from build123d import *

# Parameters (mm, degrees)
BOSS_EXTRUDE1_DEPTH   = 6.35
SKETCH2_W             = 18
SKETCH2_H             = 3
SKETCH2_W_2           = 10
SKETCH2_H_2           = 5
CUT_EXTRUDE1_DEPTH    = 148.509567486
CUT_EXTRUDE2_DEPTH    = 148.509567486
F_3_0MM_DOWEL_HOLE1_D = 3.2


with BuildPart() as part:
    # Sketch1 → Boss-Extrude1 (new body)
    with BuildSketch(Plane(origin=(0, 0, 0), x_dir=(1, 0, 0), z_dir=(0, 1, 0))):
        Polygon((64.951905284, 87.5), (-64.951905284, 87.5), (-108.253175473, 12.5), (-43.301270189, -100), (43.301270189, -100), (108.253175473, 12.5), align=None)
    extrude(amount=BOSS_EXTRUDE1_DEPTH)

    # Sketch2 → Cut-Extrude1 (cut, through all)
    with BuildSketch(Plane(origin=(0, 6.35, 0), x_dir=(1, 0, 0), z_dir=(0, 1, 0))):
        with Locations((-29, -92.2)):
            Rectangle(SKETCH2_W, SKETCH2_H)
        with Locations((29, -92.2)):
            Rectangle(SKETCH2_W, SKETCH2_H)
        Polygon((-62.146580335, 79.758965344), (-59.548504123, 78.258965344), (-68.548504123, 62.670508076), (-71.146580335, 64.170508076), align=None)
        Polygon((-97.548504123, 12.441034656), (-88.548504123, 28.029491924), (-91.146580335, 29.529491924), (-100.146580335, 13.941034656), align=None)
        Polygon((100.146580335, 13.941034656), (91.146580335, 29.529491924), (88.548504123, 28.029491924), (97.548504123, 12.441034656), align=None)
        Polygon((59.548504123, 78.258965344), (62.146580335, 79.758965344), (71.146580335, 64.170508076), (68.548504123, 62.670508076), align=None)
        with Locations((-29, -69.2)):
            Rectangle(SKETCH2_W_2, SKETCH2_H_2)
        with Locations((29, -69.2)):
            Rectangle(SKETCH2_W_2, SKETCH2_H_2)
        Polygon((79.094021451, 6.405136271), (74.094021451, 15.065390309), (69.763894432, 12.565390309), (74.763894432, 3.905136271), align=None)
        Polygon((40.763894432, 62.794863729), (45.094021451, 65.294863729), (50.094021451, 56.634609691), (45.763894432, 54.134609691), align=None)
        Polygon((-74.763894432, 3.905136271), (-69.763894432, 12.565390309), (-74.094021451, 15.065390309), (-79.094021451, 6.405136271), align=None)
        Polygon((-45.094021451, 65.294863729), (-40.763894432, 62.794863729), (-45.763894432, 54.134609691), (-50.094021451, 56.634609691), align=None)
    extrude(amount=-CUT_EXTRUDE1_DEPTH, mode=Mode.SUBTRACT)

    # Sketch4 → Cut-Extrude2 (cut, through all)
    with BuildSketch(Plane(origin=(0, 6.35, 0), x_dir=(1, 0, 0), z_dir=(0, 1, 0))):
        Polygon((35, -60.621778265), (70, 0), (35, 60.621778265), (-35, 60.621778265), (-70, 0), (-35, -60.621778265), align=None)
    extrude(amount=-CUT_EXTRUDE2_DEPTH, mode=Mode.SUBTRACT)

    # Ø3.0mm Dowel Hole1 (through all)
    with Locations(Plane(origin=(0, 6.35, 0), x_dir=(1, 0, 0), z_dir=(0, 1, 0))):
        with Locations((0, 74.060889132), (-64.138611416, -37.030444566), (64.138611416, -37.030444566)):
            Hole(F_3_0MM_DOWEL_HOLE1_D / 2)


solid = part.part
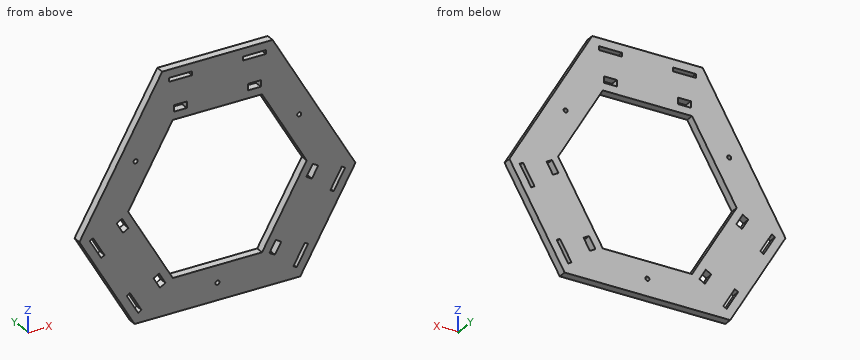
For this review, take the finished solid that the model builds, in its own axes (mm). Give positions to 0.01 mm unless a question says otherwise; leave off trailing zeros. Order: outer loops, then holes, each group sorted by start corner. A loop starts at its lowest first (then second) coordinate and runs counter-clockwise, first axis right, second up. Notation, with made-up numbers: (74.5, 42) -> (79.5, 42) arc R11 cw to (79.5, 55) -> close; hole circle Ø6 at (-34, 27). An arc over 180 degrees is marked (long way). Write item = value, one per line.
1) We need section A-A, the plane x = 9.5. Give the boundary of the cut face in (y, z), and give its area (3 significant figures).
Findings:
outline = (0, -87.5) -> (6.35, -87.5) -> (6.35, -60.62) -> (0, -60.62) -> close; (0, 60.62) -> (6.35, 60.62) -> (6.35, 100) -> (0, 100) -> close
area = 421 mm^2
2) To check wall thickness, follow L1, parallel to Z at x = 0, y = 2.5; L2, parallel to Z at x = 60.5, y = 0.75; L3, parallel to Z at x = 26, y = 3.75. State the ranges of each line that lie inside material, in increasing order. Write a range as from..to.
Findings:
L1 = -87.5..-75.66, -72.46..-60.62, 60.62..100
L2 = -87.5..-78.81, -76.61..-16.45, 16.45..70.21
L3 = -87.5..-60.62, 60.62..66.7, 71.7..90.7, 93.7..100
3) We need section B-B, the plane z = 14. Give the boundary of the cut face in (x, y), and give its area (3 significant figures).
Findings:
outline = (-92.95, 0) -> (-61.92, 0) -> (-61.92, 6.35) -> (-92.95, 6.35) -> close; (61.92, 0) -> (92.95, 0) -> (92.95, 6.35) -> (61.92, 6.35) -> close
area = 394 mm^2
4) We need section C-C, the plane y = 5. Count the separate pieces of the cut face and the enclosed holes in it, and give its area (3 significant figures).
Findings:
separate_pieces = 1
enclosed_holes = 16
area = 16,700 mm^2
5) Insertion check: pin 1 (1 mm diameter, centred on y = 3, z = 19.5, fed in from +X); pin 2 (2.5 mm diameter, centred on y = 3.5, z = 69.5, fed in from +X); pin 3 (3.5 mm diameter, centred on y = 4, z = 92, fed in from -X). Each pin has a flat end and moves straight along its axis. Give the tip position at first contact, or say it passes through.
Findings:
pin_1 = 90.07
pin_2 = 61.63
pin_3 = -48.93
